Here's how the part is built. I have some questions about the finished solid (model axes, mm). A direction names the side the tool comes from. Round coordinates to 2 decimals unless told otherwise and drop trailing zeros. Order: outer loops, then holes, each group sorted by start corner. A loop starts at its lowest first (then second) coordinate and runs counter-clockwise, first axis right, second up. Notation, with made-up numbers: (49.25, 60.25) -> (69.25, 60.25) arc R22 ccw to (69.25, 76.25) -> close; hole circle Ø10 at (-1.75, 64). An arc over 180 degrees is marked (long way). One line per item, written item: value.
```python
from build123d import *

# Parameters (mm, degrees)
F0_W      = 49
F0_H      = 22
F0_W_2    = 45
F0_H_2    = 18
F1_DEPTH  = 11
F2_W      = 49
F2_H      = 22
F3_DEPTH  = 1.4
F4_W      = 5
F4_H      = 8
F5_DEPTH  = 2
F6_R      = 1.5
F7_DEPTH  = 2
F8_W      = 3
F8_H      = 3
F9_DEPTH  = 11
F10_R     = 2.5
F11_R     = 2.5
F12_R     = 2.49999
F14_D     = 1.5
F14_DEPTH = 8
F14_TIP   = 0.4506454643
F15_SIZE  = 0.4


# Not quite as in the source:
# - a fillet or chamfer is up to 0.001 mm smaller than in the source, because OpenCascade refuses the exact size


with BuildPart() as f1:
    # F0 (on Top) → F1 (new body)
    with BuildSketch(Plane.XY):
        with Locations((22.5, 9)):
            Rectangle(F0_W, F0_H)
        with Locations((22.5, 9)):
            Rectangle(F0_W_2, F0_H_2, mode=Mode.SUBTRACT)
    extrude(amount=F1_DEPTH)

    # F2 (on face) → F3 (join)
    with BuildSketch(Plane(origin=(0, 0, 0), x_dir=(1, 0, 0), z_dir=(0, 0, -1))):
        with Locations((22.5, -9)):
            Rectangle(F2_W, F2_H)
    extrude(amount=F3_DEPTH)

    # F4 (on face) → F5 (cut, through all)
    with BuildSketch(Plane.YZ.offset(47)):
        with Locations((9, 7)):
            Rectangle(F4_W, F4_H)
    extrude(amount=-F5_DEPTH, mode=Mode.SUBTRACT)

    # F6 (on face) → F7 (cut, through all)
    with BuildSketch(Plane(origin=(0, 20, 0), x_dir=(-1, 0, 0), z_dir=(0, 1, 0))):
        with Locations((-30.5, 8)):
            Circle(F6_R)
    extrude(amount=-F7_DEPTH, mode=Mode.SUBTRACT)

    # F8 (on face) → F9 (join, through all)
    with BuildSketch(Plane.XY):
        with Locations((1.5, 1.5)):
            Rectangle(F8_W, F8_H)
        with Locations((43.5, 1.5)):
            Rectangle(F8_W, F8_H)
        with Locations((1.5, 16.5)):
            Rectangle(F8_W, F8_H)
        with Locations((43.5, 16.5)):
            Rectangle(F8_W, F8_H)
    extrude(amount=F9_DEPTH)

    # F10
    f10_edges = [f1.edges().sort_by_distance(p)[0] for p in [
        (42, 3, 5.5),
        (42, 15, 5.5),
        (3, 3, 5.5),
        (3, 15, 5.5),
    ]]
    fillet(f10_edges, radius=F10_R)

    # F11
    f11_edges = [f1.edges().sort_by_distance(p)[0] for p in [
        (47, -2, 4.8),
        (47, 20, 4.8),
        (-2, 20, 4.8),
        (-2, -2, 4.8),
    ]]
    fillet(f11_edges, radius=F11_R)

    # F12 (radius 2.5 in the source; OpenCascade refuses exactly that, so slightly less here)
    f12_edges = [f1.edges().sort_by_distance(p)[0] for p in [
        (46, 11.5, 3),
        (46, 6.5, 3),
    ]]
    fillet(f12_edges, radius=F12_R)

    # F14
    with Locations(Plane.XY.offset(11)):
        with Locations((44.5, 17.5), (44.5, 0.5), (0.5, 0.5), (0.5, 17.5)):
            Hole(F14_D / 2, depth=F14_DEPTH)
            with Locations((0, 0, -(F14_DEPTH + F14_TIP / 2))):  # 118° drill point
                Cone(0, F14_D / 2, F14_TIP, mode=Mode.SUBTRACT)

    # F15
    f15_edges = [f1.edges().sort_by_distance(p)[0] for p in [
        (-2, 9, -1.4),
        (-1.267767, -1.267767, -1.4),
        (-1.267767, 19.267767, -1.4),
        (22.5, -2, -1.4),
        (22.5, 20, -1.4),
        (46.267767, -1.267767, -1.4),
        (46.267767, 19.267767, -1.4),
        (47, 9, -1.4),
    ]]
    chamfer(f15_edges, length=F15_SIZE)


solid = f1.part
```
Q1. I want a section at C-C on x = 39. Write out the boundary of the cut face in (y, z), then the cut area to 3 significant figures.
Answers:
outline: (-2, -1) -> (-1.6, -1.4) -> (19.6, -1.4) -> (20, -1) -> (20, 11) -> (18, 11) -> (18, 0) -> (0, 0) -> (0, 11) -> (-2, 11) -> close
area: 74.6 mm2
Q2. I want a section at B-B on y = 14.25. Write out the boundary of the cut face in (x, z), then the cut area to 3 significant figures.
Answers:
outline: (-2, -1) -> (-1.6, -1.4) -> (46.6, -1.4) -> (47, -1) -> (47, 11) -> (45, 11) -> (45, 0) -> (0, 0) -> (0, 11) -> (-2, 11) -> close
area: 112 mm2
Q3. If we mould it in two halves opening along X, with no side actions, what happens to faces 1 (the face through (46.287, -1.248, 5.084)), 2 (the face through (0.48, 17.63, 2.63)), 3 (the face through (46, 6.5, 8)), 4 (the face through (-1.248, -1.287, 5.084))? For each: pulls with the +X half, pulls with the -X half, needs draft (parallel to the pull), parting line crosses it, or undercut.
Answers:
face 1: pulls with the +X half
face 2: undercut
face 3: needs draft
face 4: pulls with the -X half
Q4. I need wall thicknesses on line 1 along X through (y, z) = (17.5, 7.75); line 2 along Y through (x, z) = (17.5, 8.5); line 3 along X through (y, z) = (12, 10). Which ranges of each line are inside material? Lowest first, please.
Answers:
line 1: -2 to -0.25, 1.25 to 3, 42 to 43.75, 45.25 to 47
line 2: -2 to 0, 18 to 20
line 3: -2 to 0, 45 to 47
Q5. I want a section at A-A on x = 30.5. Write out the boundary of the cut face in (y, z), then the cut area to 3 significant figures.
Answers:
outline: (-2, -1) -> (-1.6, -1.4) -> (19.6, -1.4) -> (20, -1) -> (20, 6.5) -> (18, 6.5) -> (18, 0) -> (0, 0) -> (0, 11) -> (-2, 11) -> close; (18, 9.5) -> (20, 9.5) -> (20, 11) -> (18, 11) -> close
area: 68.6 mm2
Q6. Which directions (+Z, -Z, +X, -X, +Y, -Y) give clear straight access to the entire face, cutting with the end or side of a thin tool? Please do faces 5 (the face through (22, 9, 0)), 6 (the face through (46, 11, 4)), 7 (the face through (32, 19, 8)).
Answers:
face 5: +Z
face 6: +Z, +X
face 7: +Y
Q7. I want a section at D-D on z = 7.25. Give the number of separate pieces and of enclosed holes in the cut face, then the cut area to 3 significant figures.
Answers:
separate pieces: 2
enclosed holes: 4
area: 271 mm2
Q8. For P1, Ø2, axis at x = 45.5, z = 9, coming from the +Y side; P2, Ø8, axis at x = 27, y = 7, coming from the +Z side; P3, Ø2, axis at x = 46.5, z = 9.5, coming from the -Y side, each with a flat end and sliding along its axis, tell me the tip position at first contact or that it passes through.
Answers:
P1: y = 20
P2: z = 0
P3: y = -1.79
